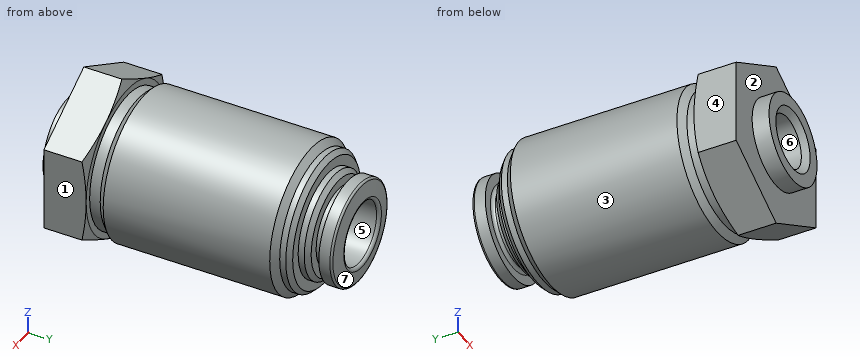
Autodesk Inventor part; units mm, degrees
ref_plane "MUTTER1_XY" through (0, 10, 0) normal (0, 1, 0) x (1, 0, 0)
ref_plane "MUTTER1_YZ" through (0, 10, 0) normal (1, 0, 0) x (0, 0, -1)
ref_plane "MUTTER1_ZX" through (0, 10, 0) normal (0, 0, -1) x (0, 1, 0)
sketch "Sketch_2" plane through (0, 0, 0) normal (0, 0, 1) x (1, 0, 0)
  line L0 (0, 0) -> (0, 28)
  line L1 (0, 28) -> (3.3, 28)
  line L2 (3.3, 28) -> (4.7347, 27.747)
  arc A0 (4.9, 27.5501) -> (4.7347, 27.747) centre (4.7, 27.5501) ccw
  line L3 (4.9, 27.5501) -> (4.9, 26.5)
  line L4 (4.9, 26.5) -> (4, 26.5)
  arc A1 (4, 26.5) -> (3.7, 26.2) centre (4, 26.2) ccw
  line L5 (3.7, 26.2) -> (3.7, 25.6)
  line L6 (3.7, 25.6) -> (4.5757, 25.6)
  line L7 (4.5757, 25.6) -> (5, 25.1757)
  line L8 (5, 25.1757) -> (5, 24.6)
  line L9 (5, 24.6) -> (5.9622, 24.6)
  line L10 (5.9622, 24.6) -> (6.3865, 24.1757)
  line L11 (6.3865, 24.1757) -> (6.3865, 23.6)
  line L12 (6.3865, 23.6) -> (7, 22.9865)
  line L13 (7, 22.9865) -> (7, 7.2135)
  line L14 (7, 7.2135) -> (6.3865, 6.6)
  line L15 (6.3865, 6.6) -> (6.3865, 5.6)
  line L16 (6.3865, 5.6) -> (7, 5.6)
  line L17 (7, 5.6) -> (8.4, 5.0904)
  line L18 (8.4, 5.0904) -> (8.4, 1.6)
  line L19 (8.4, 1.6) -> (4.2, 1.6)
  line L20 (4.2, 1.6) -> (4.2, 0)
  line L21 (4.2, 0) -> (0, 0)
  line L22 (0, 0) -> (0, 28)
revolve "Revolution1" add sketch "Sketch_2" angle 360 about axis through (0, 0, 0) along (0, -1, 0)
thread "Thread1"
sketch "Sketch_3" plane through (0, 0, 0) normal (0, 0, 1) x (1, 0, 0)
  line L0 (0, 0) -> (0, 28)
  line L1 (0, 28) -> (3.3, 28)
  arc A0 (3.3, 28) -> (3, 27.7) centre (3.3, 27.7) ccw
  line L2 (3, 27.7) -> (3, 16)
  line L3 (3, 16) -> (1.5, 16)
  line L4 (1.5, 16) -> (1.5, 12.9585)
  line L5 (1.5, 12.9585) -> (2.4585, 12)
  line L6 (2.4585, 12) -> (2.4585, 0.5415)
  line L7 (2.4585, 0.5415) -> (3, 0)
  line L8 (3, 0) -> (0, 0)
  line L9 (0, 0) -> (0, 28)
revolve "Revolution2" cut sketch "Sketch_3" angle 360 about axis through (0, 0, 0) along (0, -1, 0)
thread "Thread2"
sketch "Sketch_1" plane through (0, 5.6, 0) normal (0, 1, 0) x (1, 0, 0)
  line L0 (-13.4451, -13.8453) -> (13.2851, -13.8453)
  line L1 (13.2851, -13.8453) -> (13.2851, 13.6852)
  line L2 (13.2851, 13.6852) -> (-13.4451, 13.6852)
  line L3 (-13.4451, 13.6852) -> (-13.4451, -13.8453)
  line L4 (-7, -4.0415) -> (0, -8.0829)
  line L5 (0, -8.0829) -> (7, -4.0415)
  line L6 (7, -4.0415) -> (7, 4.0415)
  line L7 (7, 4.0415) -> (0, 8.0829)
  line L8 (0, 8.0829) -> (-7, 4.0415)
  line L9 (-7, 4.0415) -> (-7, -4.0415)
extrude "Extrusion1" cut sketch "Sketch_1" against normal blind 5.6
ref_plane "MUTTER1_XY" through (0, 10, 0) normal (0, 1, 0) x (1, 0, 0)
ref_plane "MUTTER1_YZ" through (0, 10, 0) normal (1, 0, 0) x (0, 0, -1)
ref_plane "MUTTER1_ZX" through (0, 10, 0) normal (0, 0, -1) x (0, 1, 0)
ref_plane "MUTTER2_XY" through (0, 18, 0) normal (0, 1, 0) x (1, 0, 0)
ref_plane "MUTTER2_YZ" through (0, 18, 0) normal (1, 0, 0) x (0, 0, -1)
ref_plane "MUTTER2_ZX" through (0, 18, 0) normal (0, 0, -1) x (0, 1, 0)
ref_plane "Sauger_XY" through (0, 0, 0) normal (0, 1, 0) x (1, 0, 0)
ref_plane "Sauger_YZ" through (0, 0, 0) normal (1, 0, 0) x (0, 0, -1)
ref_plane "Sauger_ZX" through (0, 0, 0) normal (0, 0, -1) x (0, 1, 0)
properties part number "189199 ESH-HA-4-QS"
The model under review builds one solid part; all positions refer to its coordinate system, in mm. Face numbers are marked on the shaded views. A direction names the side the tool comes from. Give positions to 0.01 mm unless a question says otherwise; leave off trailing zeros. Order: outer loops, then holes, each group sorted by start corner. A loop starts at its lowest first (then second) coordinate and runs counter-clockwise, first axis right, second up. Notation, with made-up numbers: M -1,73.5 L 39,73.5 A22 cw 39,99.5 Z; hole C 77.25,54.25 d10. An arc over 180 degrees is marked long. Answer in a Markdown table with one row per item. Add a question column.
1. Mouldability with a two-part tool opening along X and no side actions: class the marked faces 4, 5, 6 and 7 as released by +X, released by -X, zero draft, split by the parting line, or undercut.
2. Add section B-B on y = 19.5. State the section outline as (x, z) points.
3. For pin 1 Ø3 at (x, z) = (0.5, 0) entering from +Y; pin 2 Ø8 at (x, z) = (-4, -0.5) entering from +Y; pin 3 Ø1.5 at (y, z) = (24, -1) entering from -X; pin 4 Ø2 at (y, z) = (20.5, 2) entering from -X, all flat-tipped, find the tip position at first contact; note any pin that passes through.
4. To check wall thickness, follow line 1 along Z through (x, y) = (0, 6.5); line 2 along Z through (x, y) = (0, 14.4); line 3 along X through (y, z) = (25, 0.5). State the ranges of each line that lie inside material, in increasing order.
5. Add section A-A on y = 15. State the section outline as (x, z) points, plus the area to 3 significant figures.
6. Machinability: for the marked faces 1, 2 and 3, which of the approach directions +Z, -Z, +X, -X, +Y, -Y give a long, thin tool a straight path to every point of the face, cutting with its end or side? Answer none if there is none.
The answers:
| question | item | result |
|---|---|---|
| 1 | face 4 | released by -X |
| 1 | face 5 | undercut |
| 1 | face 6 | undercut |
| 1 | face 7 | split by the parting line |
| 2 | outline | C 0,0 d14; hole C 0,0 d6 |
| 3 | pin 1 | y = 16 |
| 3 | pin 2 | y = 28 |
| 3 | pin 3 | x = -6.67 |
| 3 | pin 4 | x = -6.93 |
| 4 | line 1 | -6.39 to -2.46, 2.46 to 6.39 |
| 4 | line 2 | -7 to -1.5, 1.5 to 7 |
| 4 | line 3 | -4.97 to -2.96, 2.96 to 4.97 |
| 5 | outline | C 0,0 d14; hole C 0,0 d3 |
| 5 | area | 147 mm2 |
| 6 | face 1 | +Z, -Z, +X, +Y, -Y |
| 6 | face 2 | -Y |
| 6 | face 3 | +Y |
